Read the model definition and answer for the solid it produces. Units are mm, in the model's axes. Face numbers are marked on the shaded views. A direction names the side the tool comes from. Coordinates: 2 decimals unless noted, no trailing zeros. Write each loop counter-clockwise with the first axis right and the second up, starting at its lowest first coordinate (ties: lowest second). Pieces come first, ordered by that corner, then holes. Notation, with made-up numbers: (51, 25) -> (73, 25) arc R10 ccw to (73, 44) -> close; hole circle Ø11 at (40, -13.75). An arc over 180 degrees is marked (long way). Answer as a JSON object with one key per item and string values. Group by question number.
(1) Flat-ended cylindrical pins translate along their axes: P1, Ø3, axis at x = -9.5, z = 3.5, coming from the -Y side; P2, Ø3, axis at x = 2.14, z = 4.7, coming from the +Y side; P3, Ø3, axis at x = 5, y = 1.5, coming from the +Z side. Find the tip coordinate at first contact, or state that the pin passes through.
(2) Find section C-C (z = 5.25). Give the vertices of the cut face in (x, y).
(3) Straight lines are drawn through the part: L1, parallel to X at y = 4, z = 4.75; L2, parallel to Z at x = -4.5, y = -1.25; L3, parallel to X at y = 3.5, z = 2.25. For each, find the intervals that lie inside material, in ascending order.
(4) Find section A-A (z = 2.25). Give the vertices of the cut face in (x, y).
(5) Find section D-D (z = 0.5). Give the vertices of the cut face in (x, y).
(6) Which of the six approach directions +Z, -Z, +X, -X, +Y, -Y give full straight-line access (tool end or side, diameter ignored) to the marked faces 1, 2 and 3?
(7) Find section B-B (x = -10). Give the vertices of the cut face in (y, z), then the cut area to 3 significant figures.
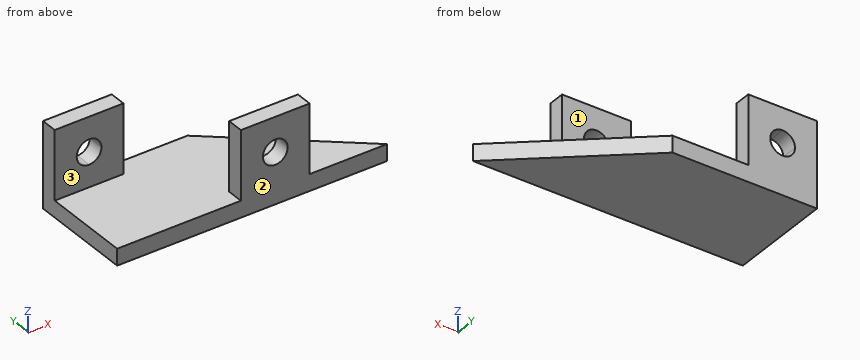
from build123d import *

# Parameters (mm, degrees)
F0_W     = 4.572
F0_H     = 1.524
F0_W_2   = 1.778
F0_H_2   = 8.128
F0_W_3   = 6.35
F1_DEPTH = 1.524
F2_W     = 6.35
F2_H     = 1.524
F3_DEPTH = 6.35
F5_DEPTH = 2.54
F6_DEPTH = 6.35
F7_R     = 1.143
F8_DEPTH = 2.54


with BuildPart() as f1:
    # F0 (on Top) → F1 (new body)
    with BuildSketch(Plane.XY):
        with Locations((3.159252, -4.064)):
            Rectangle(F0_W, F0_H)
        with Locations((-0.015748, 0.762)):
            Rectangle(F0_W_2, F0_H_2)
        Polygon((-0.904748, -3.302), (-0.904748, 4.826), (-6.111748, 4.826), (-6.111748, 3.302), (-12.461748, 3.302), (-12.461748, -4.826), (-0.904748, -4.826), align=None)
        Polygon((7.2287730873, -4.826), (12.461748, -4.826), (0.873252, 4.826), (0.873252, -3.302), (5.445252, -3.302), (5.445252, -4.826), align=None)
        with Locations((-9.286748, 4.064)):
            Rectangle(F0_W_3, F0_H)
        with Locations((-0.015748, -4.064)):
            Rectangle(F0_W_2, F0_H)
    extrude(amount=F1_DEPTH)

    # F2 (on face) → F3 (join)
    with BuildSketch(Plane.XY.offset(1.524)):
        with Locations((-9.286748, 4.064)):
            Rectangle(F2_W, F2_H)
    extrude(amount=F3_DEPTH)

    # F4 (on face) → F5 (cut)
    with BuildSketch(Plane.XZ.offset(-3.302)):
        with BuildLine():
            Line((-9.286748, 4.699), (-8.143748, 4.699))
            ThreePointArc((-8.143748, 4.699), (-8.4785249491, 5.5072230509), (-9.286748, 5.842))
            Line((-9.286748, 5.842), (-9.286748, 4.699))
        make_face()
        with BuildLine():
            Line((-10.429748, 4.699), (-9.286748, 4.699))
            Line((-9.286748, 4.699), (-9.286748, 5.842))
            ThreePointArc((-9.286748, 5.842), (-10.0949710509, 5.5072230509), (-10.429748, 4.699))
        make_face()
        with BuildLine():
            Line((-9.286748, 3.556), (-9.286748, 4.699))
            Line((-9.286748, 4.699), (-10.429748, 4.699))
            ThreePointArc((-10.429748, 4.699), (-10.0949710509, 3.8907769491), (-9.286748, 3.556))
        make_face()
        with BuildLine():
            ThreePointArc((-9.286748, 3.556), (-8.4785249491, 3.8907769491), (-8.143748, 4.699))
            Line((-8.143748, 4.699), (-9.286748, 4.699))
            Line((-9.286748, 4.699), (-9.286748, 3.556))
        make_face()
    extrude(amount=-F5_DEPTH, mode=Mode.SUBTRACT)

    # F2 (on face) → F6 (join)
    with BuildSketch(Plane.XY.offset(1.524)):
        with Locations((2.143252, -4.064)):
            Rectangle(F2_W, F2_H)
    extrude(amount=F6_DEPTH)

    # F7 (on face) → F8 (cut)
    with BuildSketch(Plane(origin=(0, -3.302, 0), x_dir=(-1, 0, 0), z_dir=(0, 1, 0))):
        with Locations((-2.143252, 4.699)):
            Circle(F7_R)
    extrude(amount=-F8_DEPTH, mode=Mode.SUBTRACT)


solid = f1.part
Results below:
{
 "1": {"P1": "stops at y = 3.3", "P2": "stops at y = -3.3", "P3": "stops at z = 1.52"},
 "2": {"outline": "(-12.46, 3.3) -> (-10.29, 3.3) -> (-10.29, 4.83) -> (-12.46, 4.83) -> close; (-8.29, 3.3) -> (-6.11, 3.3) -> (-6.11, 4.83) -> (-8.29, 4.83) -> close; (-1.03, -4.83) -> (1.14, -4.83) -> (1.14, -3.3) -> (-1.03, -3.3) -> close; (3.14, -4.83) -> (5.32, -4.83) -> (5.32, -3.3) -> (3.14, -3.3) -> close"},
 "3": {"L1": "x = -12.46 to -10.43, -8.14 to -6.11", "L2": "z = 0 to 1.52", "L3": "x = -12.46 to -6.11"},
 "4": {"outline": "(-12.46, 3.3) -> (-6.11, 3.3) -> (-6.11, 4.83) -> (-12.46, 4.83) -> close; (-1.03, -4.83) -> (5.32, -4.83) -> (5.32, -3.3) -> (-1.03, -3.3) -> close"},
 "5": {"outline": "(-12.46, -4.83) -> (12.46, -4.83) -> (0.87, 4.83) -> (-12.46, 4.83) -> close"},
 "6": {"face 1": "+Z, +X, -X, +Y", "face 2": "+Z, -Z, +X, -X, -Y", "face 3": "+Z, +X, -X, -Y"},
 "7": {"outline": "(-4.83, 0) -> (4.83, 0) -> (4.83, 3.81) -> (3.3, 3.81) -> (3.3, 1.52) -> (-4.83, 1.52) -> close; (3.3, 5.59) -> (4.83, 5.59) -> (4.83, 7.87) -> (3.3, 7.87) -> close", "area": "21.7 mm2"}
}
